Check sheet for the modelled part. Datum: model origin and axes. Units: mm. A direction names the side the tool comes from. Round coordinates to 2 decimals unless told otherwise and drop trailing zeros. Write each loop counter-clockwise with the first axis right and the second up, starting at its lowest first coordinate (ties: lowest second). Pieces come first, ordered by that corner, then holes. Notation, with made-up numbers: (-33, 7.5) - (-17, 7.5) arc R14 ccw to (-17, 29.5) - close; hole circle Ø3 at (85.25, 41). An arc over 180 degrees is marked (long way). Answer as a JSON object with one key per item and string values. Group by question number.
Item 1: Thickness scan on line 1 (Z direction, x = -4, y = -8); line 2 (X direction, y = 0.25, z = 74.5); line 3 (Z direction, x = 5.75, y = 3.5). Record the ranges inside material, lowest first.
Item 2: Sectioned sample at A-A on x = 0. Record the boundary of the cut face in (y, z).
Item 3: Gauge pin test, flat ends, axial feed: P1, Ø1.5, axis at y = -5, z = 27.5, coming from the +X side; P2, Ø12, axis at y = 7.5, z = 70, coming from the -X side; P3, Ø5, axis at y = -3, z = 37.5, coming from the +X side; P4, Ø2, axis at x = 5, y = 4.5, coming from the -Z side. Record the tip position at first contact, or that the pin passes through.
Item 4: Set-up check for faces 1 (the flat face through (0, 0, 80)), 2 (the flat face through (0, -7.3, 20)): record each of +Z, -Z, +X, -X, +Y, -Y from which the full face is reachable in a straight line by a thin tool's end or side.
Item 5: Sectioned sample at C-C on z = 6. Record the boundary of the cut face in (x, y).
```python
from build123d import *

# Parameters (mm, degrees)
ESBO_O1_R                = 10
RESSALTO_EXTRUS_O1_DEPTH = 20
ESBO_O2_R                = 7
RESSALTO_EXTRUS_O2_DEPTH = 3
ESBO_O3_R                = 5
RESSALTO_EXTRUS_O3_DEPTH = 57
CHANFRO1_SIZE            = 1
CHANFRO2_SIZE            = 1
CHANFRO3_SIZE            = 1
ESBO_O5_R                = 1.5


with BuildPart() as part:
    # Esboço1 → Ressalto-extrusão1 (new body)
    with BuildSketch(Plane.XY):
        Circle(ESBO_O1_R)
    extrude(amount=RESSALTO_EXTRUS_O1_DEPTH)

    # Esboço2 → Ressalto-extrusão2 (add)
    with BuildSketch(Plane.XY.offset(20)):
        Circle(ESBO_O2_R)
    extrude(amount=RESSALTO_EXTRUS_O2_DEPTH)

    # Esboço3 → Ressalto-extrusão3 (add)
    with BuildSketch(Plane.XY.offset(23)):
        with Locations(Location((0, 0, 0), (0, 0, 180))):
            Circle(ESBO_O3_R)
    extrude(amount=RESSALTO_EXTRUS_O3_DEPTH)

    # Chanfro1
    chanfro1_edges = [part.edges().sort_by_distance(p)[0] for p in [
        (-10, 0, 0),
    ]]
    chamfer(chanfro1_edges, length=CHANFRO1_SIZE)

    # Chanfro2
    chanfro2_edges = [part.edges().sort_by_distance(p)[0] for p in [
        (-10, 0, 20),
    ]]
    chamfer(chanfro2_edges, length=CHANFRO2_SIZE)

    # Chanfro3
    chanfro3_edges = [part.edges().sort_by_distance(p)[0] for p in [
        (5, 0, 80),
    ]]
    chamfer(chanfro3_edges, length=CHANFRO3_SIZE)

    # Varredura de corte1: sweep along a path in Esboço7
    with BuildLine(Plane.XY.offset(30.5)) as varredura_de_corte1_path:
        CenterArc((0, 0), 5, 0, 360)
    # Esboço5 → Varredura de corte1 (sweep, cut)
    with BuildSketch(Plane(origin=(0, 0, 0), x_dir=(1, 0, 0), z_dir=(0, 1, 0))):
        with Locations((-5, -30.5)):
            Circle(ESBO_O5_R)
    sweep(path=varredura_de_corte1_path.line, mode=Mode.SUBTRACT)


solid = part.part
```
Completed:
{
 "1": {"line 1": "0 to 20", "line 2": "-4.99 to 4.99", "line 3": "0 to 23"},
 "2": {"outline": "(-10, 1) - (-9, 0) - (9, 0) - (10, 1) - (10, 19) - (9, 20) - (7, 20) - (7, 23) - (5, 23) - (5, 29) arc R1.5 cw to (5, 32) - (5, 79) - (4, 80) - (-4, 80) - (-5, 79) - (-5, 32) arc R1.5 cw to (-5, 29) - (-5, 23) - (-7, 23) - (-7, 20) - (-9, 20) - (-10, 19) - close"},
 "3": {"P1": "x = 2.63", "P2": "x = -4.77", "P3": "x = 4.97", "P4": "z = 0"},
 "4": {"face 1": "+Z, +X, -X, +Y, -Y", "face 2": "+Z"},
 "5": {"outline": "circle Ø20 at (0, 0)"}
}
